Print and shaded views of the part. All mm, measured from the part's lowest x, y and z. A direction names the side the tool comes from. Give positions to 0.01 mm unless a question says otherwise; leave off trailing zeros. Order: outer loops, then holes, each group sorted by start corner. A loop starts at its lowest first (then second) coordinate and runs counter-clockwise, first axis right, second up. Notation, with made-up numbers: (61.25, 48.5) -> (97.25, 48.5) arc R6 ccw to (97.25, 56.5) -> close; hole circle Ø10 at (76.5, 48). An arc over 180 degrees is marked (long way). One line per question, with ' | ' between items. Start each with the question number.
(1) Pull direction Z, two halves, no side cores. Call the marked faces 1, 2, 3 and 4: +Z half, -Z half, draft (parallel to the pull), parting line (faces both ways), or undercut.
(2) Pin check, flat tips, straight feed: pin 1 Ø2.5 at (x, y) = (16.5, 28) entering from +Z; pin 2 Ø6 at (x, z) = (4, 65.5) entering from +Y; pin 3 Ø14.5 at (x, z) = (9, 45.5) entering from +Y; pin 4 Ø2.5 at (x, z) = (16, 47.5) entering from -Y. Stop position of each tip, or through.
(3) Cut at A-A (y = 16). Give the cut face in (x, z), then the cut area to 3 significant figures.
(4) Drill centre lines: L1, parallel to Z at x = 13, y = 1; L2, parallel to Z at x = 7, y = 20; L3, parallel to Z at x = 27, y = 17. Where is each one in solid material? Low to high. Write a range as from..to.
(5) Cut at C-C (z = 47.5). Give the cut face in (x, y).
(6) Which spindle directions (+Z, -Z, +X, -X, +Y, -Y) get a long thin tool onto all of the face, cutting with end or side? Do the marked faces 5, 6 and 7. Say none if no direction does.
(7) Cut at D-D (y = 3). Give the number of separate pieces and of enclosed holes in the cut face, then the cut area to 3 significant figures.
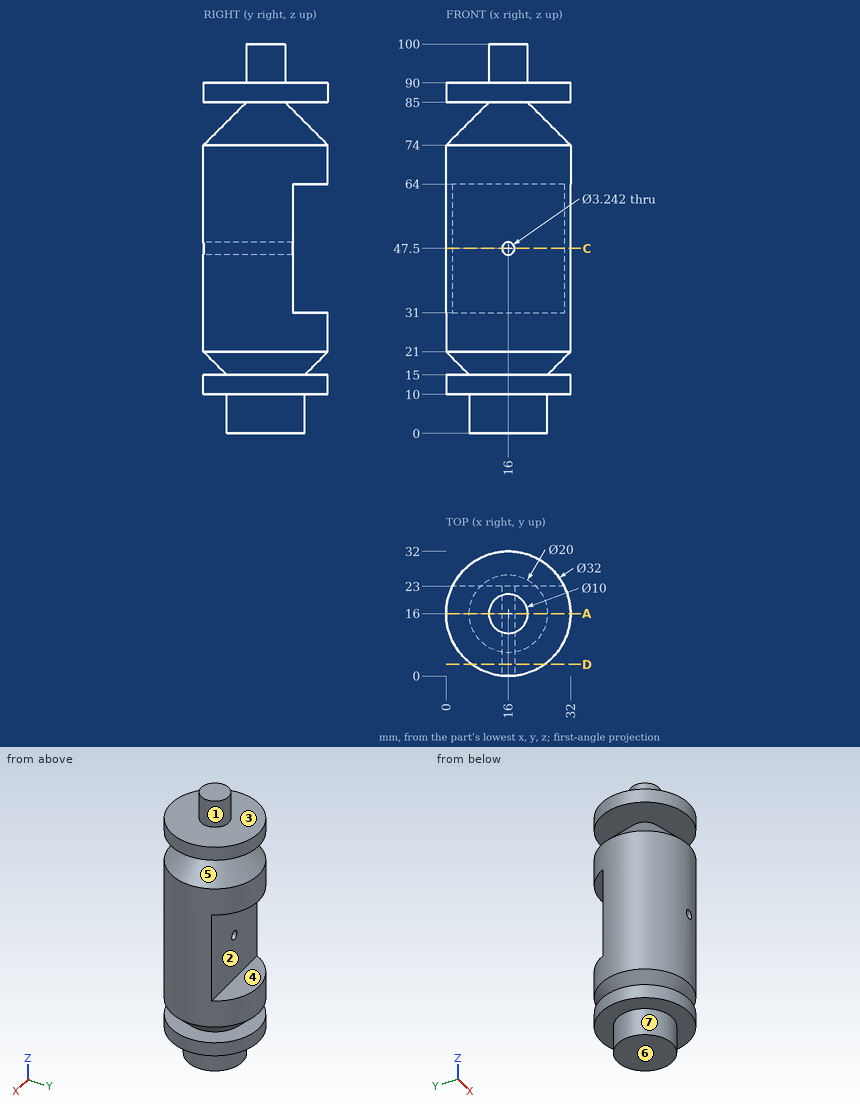
Result set:
1) face 1: draft | face 2: undercut | face 3: +Z half | face 4: undercut
2) pin 1: stops at z = 90 | pin 2: stops at y = 29.23 | pin 3: stops at y = 23 | pin 4: passes through
3) outline: (0, 10) -> (6, 10) -> (6, 0) -> (26, 0) -> (26, 10) -> (32, 10) -> (32, 15) -> (26, 15) -> (32, 21) -> (32, 74) -> (21, 85) -> (32, 85) -> (32, 90) -> (21, 90) -> (21, 100) -> (11, 100) -> (11, 90) -> (0, 90) -> (0, 85) -> (11, 85) -> (0, 74) -> (0, 21) -> (6, 15) -> (0, 15) -> close; hole circle Ø3.24 at (16, 47.5) | area: 2,690 mm2
4) L1: z = 10..15, 20.3..74.7, 85..90 | L2: z = 0..80.15, 85..90 | L3: z = 10..15, 16.05..78.95, 85..90
5) outline: (1.61, 23) arc R16 ccw to (14.38, 0.08) -> (14.38, 23) -> close; (17.62, 0.08) arc R16 ccw to (30.39, 23) -> (17.62, 23) -> close
6) face 5: none | face 6: -Z, +X, -X, +Y, -Y | face 7: -Z
7) separate pieces: 3 | enclosed holes: 1 | area: 1,240 mm2
